```python
from build123d import *

# Parameters (mm, degrees)
F1_DEPTH = 12.7
F2_DEPTH = 50.8
F3_W     = 31.75
F3_H     = 25.4
F3_R     = 6.35
F4_DEPTH = 12.7


with BuildPart() as f1:
    # F0 (on Top) → F1 (new body)
    with BuildSketch(Plane.XY):
        with BuildLine():
            Line((-38.1, -31.75), (38.1, -31.75))
            Line((38.1, -31.75), (38.1, 31.75))
            Line((38.1, 31.75), (-38.1, 31.75))
            ThreePointArc((-38.1, 31.75), (-15.64936, 22.45064), (-6.35, 0))
            ThreePointArc((-6.35, 0), (-15.64936, -22.45064), (-38.1, -31.75))
        make_face()
        with BuildLine():
            ThreePointArc((-38.1, 31.75), (-69.85, 0), (-38.1, -31.75))
            Line((-38.1, -31.75), (-38.1, -12.7))
            ThreePointArc((-38.1, -12.7), (-50.8, 0), (-38.1, 12.7))
            Line((-38.1, 12.7), (-38.1, 31.75))
        make_face()
    extrude(amount=F1_DEPTH)

    # F0 (on Top) → F2 (join)
    with BuildSketch(Plane.XY):
        with BuildLine():
            Line((-38.1, -12.7), (-38.1, -31.75))
            ThreePointArc((-38.1, -31.75), (-15.64936, -22.45064), (-6.35, 0))
            ThreePointArc((-6.35, 0), (-15.64936, 22.45064), (-38.1, 31.75))
            Line((-38.1, 31.75), (-38.1, 12.7))
            ThreePointArc((-38.1, 12.7), (-29.119744, 8.980256), (-25.4, 0))
            ThreePointArc((-25.4, 0), (-29.119744, -8.980256), (-38.1, -12.7))
        make_face()
        with BuildLine():
            ThreePointArc((-38.1, 31.75), (-69.85, 0), (-38.1, -31.75))
            Line((-38.1, -31.75), (-38.1, -12.7))
            ThreePointArc((-38.1, -12.7), (-50.8, 0), (-38.1, 12.7))
            Line((-38.1, 12.7), (-38.1, 31.75))
        make_face()
    extrude(amount=F2_DEPTH)

    # F3 (on face) → F4 (join)
    with BuildSketch(Plane.YZ.offset(38.1)):
        Polygon((31.75, 12.7), (-31.75, 12.7), (-31.75, 0), (0, 0), (31.75, 0), align=None)
        with Locations((-15.875, -12.7)):
            Rectangle(F3_W, F3_H)
        with Locations((-12.7, -12.7)):
            Circle(F3_R, mode=Mode.SUBTRACT)
        with Locations((15.875, -12.7)):
            Rectangle(F3_W, F3_H)
        with Locations((12.7, -12.7)):
            Circle(F3_R, mode=Mode.SUBTRACT)
    extrude(amount=-F4_DEPTH)


solid = f1.part
```
CAD build for the part. Positions are in the model's coordinates, mm. A direction names the side the tool comes from. Coordinates: 2 decimals unless noted, no trailing zeros. Loops run counter-clockwise (first coordinate to the right, second up) from the corner with the lowest first, then second, coordinate; pieces in that order, holes last. Notation, with made-up numbers: (20, 10.25) - (25, 10.25) arc R23 cw to (25, 47.25) - close; hole circle Ø4 at (81.5, -0.5). An arc over 180 degrees is marked (long way). Return JSON: item names as keys, results as strings.
1. Mould opens along Z. For faces 1 (the flat face through (38.1, 0, -7)), 2 (the flat face through (32, 0, -25.4)), 3 (the cylindrical face through (31.84, -14.08, -18.9)) say: released by +Z, released by -Z, zero draft, split by the parting line, or undercut.
Result:
{"face 1": "zero draft", "face 2": "released by -Z", "face 3": "undercut"}
2. Band-saw the part on D-D (z = 23.5). Give the cut face in (x, y).
Result:
{"outline": "(-38.1, -31.75) arc R31.75 ccw to (-6.35, 0) arc R31.75 ccw to (-38.1, 31.75) arc R31.75 ccw to start; hole circle Ø25.4 at (-38.1, 0)"}
3. Band-saw the part on B-B (x = -27). Give the cut face in (y, z), and give its area (3 significant figures).
Result:
{"outline": "(-31.75, 0) - (-6.17, 0) - (-6.17, 50.8) - (-29.75, 50.8) - (-29.75, 12.7) - (-31.75, 12.7) - close; (6.17, 0) - (31.75, 0) - (31.75, 12.7) - (29.75, 12.7) - (29.75, 50.8) - (6.17, 50.8) - close", "area": "2,450 mm2"}
4. 3-axis set-ups, long thin cutter, end or side, ignore diameter. For faces 4 (the flat face through (-23, 0, 0)), 5 (the cylindrical face through (31.84, 7.66, -16.56)): which of +Z, -Z, +X, -X, +Y, -Y reach the whole face in a straight line?
Result:
{"face 4": "-Z, -X, +Y, -Y", "face 5": "+X, -X"}
5. Band-saw the part on A-A (z = -12.7). Give the cut face in (x, y), and give its area (3 significant figures).
Result:
{"outline": "(25.4, -31.75) - (38.1, -31.75) - (38.1, -19.05) - (25.4, -19.05) - close; (25.4, -6.35) - (38.1, -6.35) - (38.1, 6.35) - (25.4, 6.35) - close; (25.4, 19.05) - (38.1, 19.05) - (38.1, 31.75) - (25.4, 31.75) - close", "area": "484 mm2"}
6. Probe L1, parallel to Z at x = 33.5, y = -12.7; L2, parallel to Y at x = 29, z = -12; L3, parallel to X at y = 13.5, z = -20. List the from-to ranges inside material, lowest first. Write a range as from..to.
Result:
{"L1": "z = -25.4..-19.05, -6.35..12.7", "L2": "y = -31.75..-19.01, -6.39..6.39, 19.01..31.75", "L3": "x = 25.4..38.1"}
7. Band-saw the part on C-C (y = -9). Give the cut face in (x, z).
Result:
{"outline": "(-68.55, 0) - (-47.06, 0) - (-47.06, 50.8) - (-68.55, 50.8) - close; (-29.14, 0) - (25.4, 0) - (25.4, -7.54) - (38.1, -7.54) - (38.1, 12.7) - (-7.65, 12.7) - (-7.65, 50.8) - (-29.14, 50.8) - close; (25.4, -25.4) - (38.1, -25.4) - (38.1, -17.86) - (25.4, -17.86) - close"}
8. Drop flat-ended pins along their axis: pin 1 (12 mm diameter, centred on x = 13.5, z = -13.5, fed in from +Y); pin 2 (12 mm diameter, centred on y = 9, z = 24, fed in from -X); pin 3 (12 mm diameter, centred on x = 20, y = 24, fed in from +Z); pin 4 (16.5 mm diameter, centred on y = -12.7, z = -12.7, fed in from +X). Give the stop position or say it passes through.
Result:
{"pin 1": "passes through", "pin 2": "stops at x = -69.71", "pin 3": "stops at z = 12.7", "pin 4": "stops at x = 38.1"}
